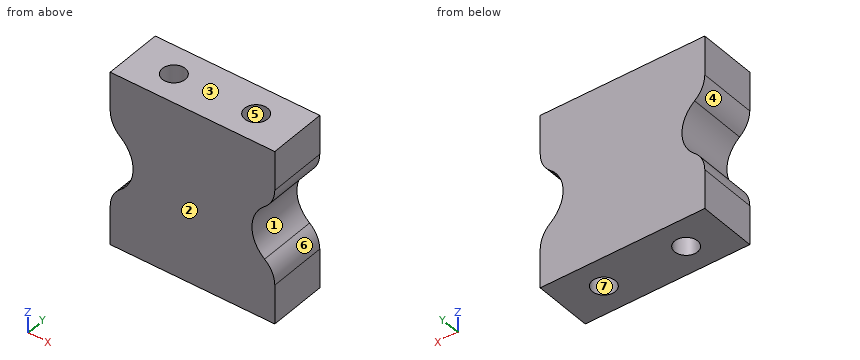
from build123d import *

# Parameters (mm, degrees)
SKETCH1_W           = 18
SKETCH1_H           = 6.35
BOSS_EXTRUDE1_DEPTH = 19.05
CUT_EXTRUDE1_DEPTH  = 7.35
SKETCH3_R           = 1.25
CUT_EXTRUDE2_DEPTH  = 5
FILLET2_R           = 3


with BuildPart() as part:
    # Sketch1 → Boss-Extrude1 (new body)
    with BuildSketch(Plane.XY):
        with Locations((9, 3.175)):
            Rectangle(SKETCH1_W, SKETCH1_H)
    extrude(amount=BOSS_EXTRUDE1_DEPTH)

    # Sketch2 → Cut-Extrude1 (cut, through all)
    with BuildSketch(Plane(origin=(0, 6.35, 0), x_dir=(1, 0, 0), z_dir=(0, 1, 0))):
        with BuildLine():
            Line((18, -6), (18, -13.05))
            ThreePointArc((18, -13.05), (15.5, -9.525), (18, -6))
        make_face()
        with BuildLine():
            Line((0, -6), (0, -13.05))
            ThreePointArc((0, -13.05), (2.5, -9.525), (0, -6))
        make_face()
    extrude(amount=-CUT_EXTRUDE1_DEPTH, mode=Mode.SUBTRACT)

    # Sketch3 → Cut-Extrude2 (cut)
    with BuildSketch(Plane(origin=(0, 0, 0), x_dir=(-1, 0, 0), z_dir=(0, 0, -1))):
        with Locations((-13.5, 3.175)):
            Circle(SKETCH3_R)
        with Locations((-4.5, 3.175)):
            Circle(SKETCH3_R)
    cut_extrude2 = extrude(amount=-CUT_EXTRUDE2_DEPTH, mode=Mode.SUBTRACT)

    # Mirror1: Cut-Extrude2 across plane
    add(cut_extrude2.mirror(Plane(origin=(0, 0, 9.525), x_dir=(1, 0, 0), z_dir=(0, 0, -1))), mode=Mode.SUBTRACT)

    # Fillet2
    fillet2_edges = [part.edges().sort_by_distance(p)[0] for p in [
        (18, 3.175, 13.05),
        (18, 3.175, 6),
        (0, 3.175, 6),
        (0, 3.175, 13.05),
    ]]
    fillet(fillet2_edges, radius=FILLET2_R)


solid = part.part
Model file for the job. Use its own axes, mm. Face numbers are marked on the shaded views. A direction names the side the tool comes from. Give positions to 0.01 mm unless a question says otherwise; leave off trailing zeros. Order: outer loops, then holes, each group sorted by start corner. A loop starts at its lowest first (then second) coordinate and runs counter-clockwise, first axis right, second up. Notation, with made-up numbers: (-17, -6) - (3, -6) arc R16 ccw to (3, 12) - close; hole circle Ø5 at (-37.5, -30.75). An arc over 180 degrees is marked (long way). Return JSON: item names as keys, results as strings.
1) Cut at D-D, the plane z = 12. Give the cut face in (x, y), plus the area to 3 significant figures.
Geometry says:
{"outline": "(1.56, 0) - (16.44, 0) - (16.44, 6.35) - (1.56, 6.35) - close", "area": "94.5 mm²"}
2) Cut at A-A, the plane y = 5.5. Give the cut face in (x, z) (3 decimals), plus the area to 3 significant figures.
Geometry says:
{"outline": "(0, 0) - (18, 0) - (18, 4.288) arc R3 ccw to (16.886, 6.621) arc R3.735 cw to (16.886, 12.429) arc R3 ccw to (18, 14.762) - (18, 19.05) - (0, 19.05) - (0, 14.762) arc R3 ccw to (1.114, 12.429) arc R3.735 cw to (1.114, 6.621) arc R3 ccw to (0, 4.288) - close", "area": "316 mm²"}
3) Probe line 1 (X direction, y = 3.25, z = 3.75); line 2 (Y direction, x = 4.5, z = 17.1) (3 decimals); line 3 (Z direction, x = 16.5, y = 2.75). List the from-to ranges inside material, lowest first. Write a range as from..to.
Geometry says:
{"line 1": "0..3.25, 5.75..12.25, 14.75..18", "line 2": "0..1.925, 4.425..6.35", "line 3": "0..6.98, 12.07..19.05"}
4) 3-axis set-ups, long thin cutter, end or side, ignore diameter. For the marked faces 4, 5, 6 and 7: which of +Z, -Z, +X, -X, +Y, -Y reach the whole face in a straight line?
Geometry says:
{"face 4": "-X, +Y, -Y", "face 5": "+Z", "face 6": "+X, +Y, -Y", "face 7": "-Z"}
5) Flat gauge pins, fed straight in: P1, Ø1.5, axis at y = 1.5, z = 8, coming from the +X side; P2, Ø3, axis at y = 2, z = 13, coming from the -X side; P3, Ø2, axis at x = 4.5, y = 3.175, coming from the -Z side. Where does each tip first touch, or does it go through?
Geometry says:
{"P1": "x = 16.27", "P2": "x = 0.01", "P3": "z = 5"}
6) Cut at C-C, the plane z = 14.5. Give the cut face in (x, y) (3 decimals), plus the area to 3 significant figures.
Geometry says:
{"outline": "(0.011, 0) - (17.989, 0) - (17.989, 6.35) - (0.011, 6.35) - close; hole circle Ø2.5 at (4.5, 3.175); hole circle Ø2.5 at (13.5, 3.175)", "area": "104 mm²"}
7) Cut at B-B, the plane x = 4.5. Give the cut face in (y, z) (3 decimals), plus the area to 3 significant figures.
Geometry says:
{"outline": "(0, 0) - (1.925, 0) - (1.925, 5) - (4.425, 5) - (4.425, 0) - (6.35, 0) - (6.35, 19.05) - (4.425, 19.05) - (4.425, 14.05) - (1.925, 14.05) - (1.925, 19.05) - (0, 19.05) - close", "area": "96.0 mm²"}
8) Pull direction Z, two halves, no side cores. Call the marked faces 1, 2 and 3: pulls with the +Z half, pulls with the -Z half, needs draft (parallel to the pull), parting line crosses it, or undercut.
Geometry says:
{"face 1": "undercut", "face 2": "needs draft", "face 3": "pulls with the +Z half"}
